from build123d import *

# Parameters (mm, degrees)
F1_DEPTH = 76.2


with BuildPart() as f1:
    # F0 (on Front) → F1 (new body)
    with BuildSketch(Plane.XZ):
        with BuildLine():
            Line((12.712441, 19.624272), (-21.695151, 19.624272))
            ThreePointArc((-21.695151, 19.624272), (-67.590624, 33.663258), (-40.246621, -5.780285))
            Line((-40.246621, -5.780285), (-40.727737, -31.175728))
            Line((-40.727737, -31.175728), (12.712441, -31.175728))
            ThreePointArc((12.712441, -31.175728), (38.112441, -5.775728), (12.712441, 19.624272))
        make_face()
    extrude(amount=F1_DEPTH)


solid = f1.part
Input: part model. Units: mm. Frame: model coordinates. A direction names the side the tool comes from. Coordinates: 2 decimals unless noted, no trailing zeros. Order: outer loops, then holes, each group sorted by start corner. A loop starts at its lowest first (then second) coordinate and runs counter-clockwise, first axis right, second up. Notation, with made-up numbers: M 34,-12.5 L 44,-12.5 A9 cw 44,3.5 Z; hole C 41.5,71 d5. An arc over 180 degrees is marked long. Write item = value, one per line. Start each with the question number.
(1) First-contact query: P1, Ø5, axis at y = -48.5, z = 25.5, coming from the +X side; P2, Ø5, axis at x = -36, y = -32, coming from the +Z side; P3, Ø17, axis at x = 2.5, y = -39, coming from the +Z side. Flat tips, straight axial feed; report the tip coordinate or a pass-through.
(2) Section C-C on z = -14. Output: boundary loops of the cut face in (x, y), and give its area (3 significant figures).
(3) Line query: line 1 along Z through (x, y) = (-13, -32); line 2 along Z through (x, y) = (-28, -53); line 3 along X through (y, z) = (-22, 24.5). Output: solid intervals per line, ascending. Write a range as [from, to].
(4) Reachability of faces 1 (the flat face through (-18, 0, 7)), 2 (the flat face through (-4, -38, 19.624)) from +Z, -Z, +X, -X, +Y, -Y: full face, straight path, thin tool, end or side. Return the list, or none.
(5) Section A-A on y = -16.5. Output: boundary loops of the cut face in (x, z), and give its area (3 significant figures).
(6) Section B-B on x = -15. Output: boundary loops of the cut face in (y, z).
Result set:
q1.P1 = -22.05
q1.P2 = 42.59
q1.P3 = 19.62
q2.outline = M -40.4,-76.2 L 36.74,-76.2 L 36.74,0 L -40.4,0 Z
q2.area = 5,880 mm²
q3.line_1 = [-31.18, 19.62]
q3.line_2 = [-31.18, 35.45]
q3.line_3 = [-71.8, -22.35]
q4.face_1 = +Z, -Z, +X, -X, +Y
q4.face_2 = +Z, +X, +Y, -Y
q5.outline = M -40.73,-31.18 L 12.71,-31.18 A25.4 ccw 12.71,19.62 L -21.7,19.62 A25.4 ccw long -40.25,-5.78 Z
q5.area = 5,380 mm²
q6.outline = M -76.2,-31.18 L 0,-31.18 L 0,19.62 L -76.2,19.62 Z
